Here's how the part is built. I have some questions about the finished solid (model axes, mm). A direction names the side the tool comes from. Round coordinates to 2 decimals unless told otherwise and drop trailing zeros. Order: outer loops, then holes, each group sorted by start corner. A loop starts at its lowest first (then second) coordinate and runs counter-clockwise, first axis right, second up. Notation, with made-up numbers: (-15, 17.5) -> (37, 17.5) arc R26 cw to (37, 55.5) -> close; hole circle Ø6 at (6, 29). An arc over 180 degrees is marked (long way). One line per item, written item: value.
```python
from build123d import *

# Parameters (mm, degrees)
SKETCH_W        = 73
SKETCH_H        = 24
PAD_DEPTH       = 40
SKETCH001_W     = 71.020102
SKETCH001_H     = 22.020102
POCKET_DEPTH    = 39
POCKET001_DEPTH = 6
CHAMFER_SIZE    = 1
FILLET_R        = 3
FILLET001_R     = 5
CHAMFER001_SIZE = 0.7


with BuildPart() as part:
    # Sketch → Pad (new body)
    with BuildSketch(Plane.XY):
        with Locations((36.5, 12)):
            Rectangle(SKETCH_W, SKETCH_H)
    extrude(amount=PAD_DEPTH)

    # Sketch001 (on Face6 of Pad) → Pocket (cut)
    with BuildSketch(Plane.XY.offset(40)):
        with Locations((36.5, 12)):
            Rectangle(SKETCH001_W, SKETCH001_H)
    extrude(amount=-POCKET_DEPTH, mode=Mode.SUBTRACT)

    # Sketch002 (on Face5 of Pocket) → Pocket001 (cut)
    with BuildSketch(Plane.XY.offset(40)):
        Polygon((0, 23.010051), (0.989949, 23.010051), (0.989949, 0.989949), (72.010051, 0.989949), (72.010051, 23.010051), (73, 23.010051), (73, 0), (0, 0), align=None)
    extrude(amount=-POCKET001_DEPTH, mode=Mode.SUBTRACT)

    # Chamfer
    chamfer_edges = [part.edges().sort_by_distance(p)[0] for p in [
        (36.5, 23.010051, 1),
        (72.010051, 12, 1),
        (36.5, 0.989949, 1),
        (0.989949, 12, 1),
    ]]
    chamfer(chamfer_edges, length=CHAMFER_SIZE)

    # Fillet
    fillet_edges = [part.edges().sort_by_distance(p)[0] for p in [
        (0, 23.505025, 40),
        (73, 23.505025, 40),
    ]]
    fillet(fillet_edges, radius=FILLET_R)

    # Fillet001
    fillet001_edges = [part.edges().sort_by_distance(p)[0] for p in [
        (0.494975, 23.010051, 34),
        (72.505025, 23.010051, 34),
    ]]
    fillet(fillet001_edges, radius=FILLET001_R)

    # Chamfer001
    chamfer001_edges = [part.edges().sort_by_distance(p)[0] for p in [
        (0, 0, 17),
        (73, 0, 17),
    ]]
    chamfer(chamfer001_edges, length=CHAMFER001_SIZE)


solid = part.part
```
Q1. I want a section at A-A on z = 32. Write out the boundary of the cut face in (x, y).
Answers:
outline: (0, 0.7) -> (0.7, 0) -> (72.3, 0) -> (73, 0.7) -> (73, 24) -> (0, 24) -> close; hole (0.99, 0.99) -> (72.01, 0.99) -> (72.01, 23.01) -> (0.99, 23.01) -> close
Q2. For P1, Ø10, axis at x = 34, y = 15, coming from the +Z side; P2, Ø10, axis at x = 10.5, y = 16, coming from the -Z side, each with a flat end and sliding along its axis, tell me the tip position at first contact or that it passes through.
Answers:
P1: z = 1
P2: z = 0
Q3. I want a section at B-B on x = 10.5. Write out the boundary of the cut face in (y, z), then the cut area to 3 significant figures.
Answers:
outline: (0, 0) -> (24, 0) -> (24, 40) -> (23.01, 40) -> (23.01, 2) -> (22.01, 1) -> (1.99, 1) -> (0.99, 2) -> (0.99, 34) -> (0, 34) -> close
area: 96.3 mm2
Q4. If we mould it in two halves opening along X, with no side actions, what happens to faces 4 (the face through (0.86, 23.46, 39.1)), 5 (the face through (0.99, 12, 21)), 6 (the face through (36, 0, 17))? For each: pulls with the +X half, pulls with the -X half, needs draft (parallel to the pull), parting line crosses it, or undercut.
Answers:
face 4: pulls with the -X half
face 5: undercut
face 6: needs draft
Q5. I want a section at C-C on y = 13.25. Write out the boundary of the cut face in (x, z), then the cut area to 3 significant figures.
Answers:
outline: (0, 0) -> (73, 0) -> (73, 34) -> (72.01, 34) -> (72.01, 2) -> (71.01, 1) -> (1.99, 1) -> (0.99, 2) -> (0.99, 34) -> (0, 34) -> close
area: 139 mm2
Q6. I need wall thicknesses on line 1 along X through (y, z) = (15, 30); line 2 along Y through (x, z) = (70, 24.5); line 3 along Z through (x, y) = (35, 5.25). Which ranges of each line are inside material? Lowest first, please.
Answers:
line 1: 0 to 0.99, 72.01 to 73
line 2: 0 to 0.99, 23.01 to 24
line 3: 0 to 1
Q7. Which directions (+Z, -Z, +X, -X, +Y, -Y) give clear straight access to the entire face, cutting with the end or side of a thin tool? Please do faces 1 (the face through (36.7, 0.4, 34)), 2 (the face through (73, 12, 18)), 3 (the face through (72.01, 12, 21)).
Answers:
face 1: +Z, +X, -X, -Y
face 2: +Z, -Z, +X, +Y, -Y
face 3: +Z
